Input: dimensioned drawing with shaded views. Units: mm. Origin: part minimum x, y, z. Give positions to 0.01 mm unless a question says otherwise; leave off trailing zeros. Write each loop counter-clockwise with the first axis right and the second up, starting at its lowest first coordinate (ties: lowest second). Pieces come first, ordered by that corner, then holes. Notation, with made-up numbers: M 89.25,-9 L 143.25,-9 A26 cw 143.25,29 Z; hole C 46,-32 d8. An arc over 180 degrees is marked long. Answer as a JSON object with one key per item and string values.
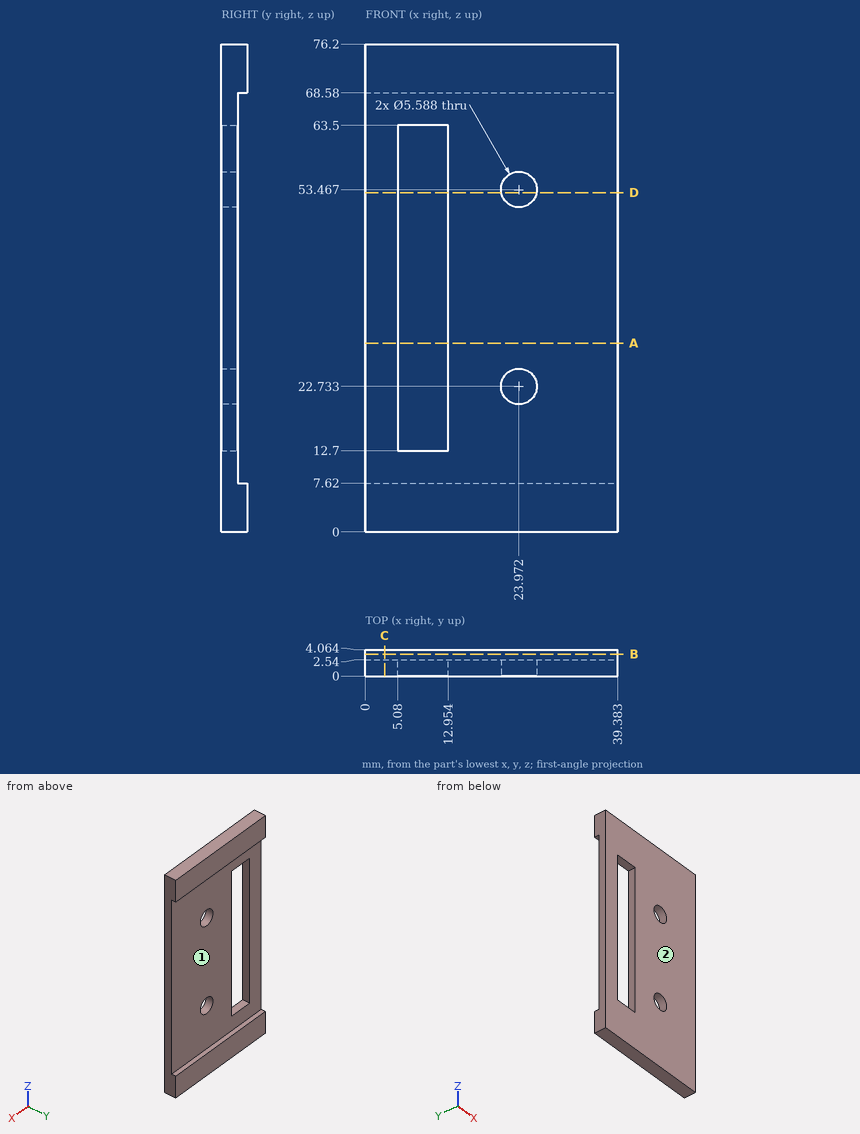
1) Cut plane D-D on z = 53. Return loops of the section in (x, y).
Geometry check:
{"outline": "M 0,0 L 5.08,0 L 5.08,2.54 L 0,2.54 Z; M 12.95,0 L 21.22,0 L 21.22,2.54 L 12.95,2.54 Z; M 26.73,0 L 39.38,0 L 39.38,2.54 L 26.73,2.54 Z"}
2) Contact query for flat-ended pins moving along their axis: P1, Ø6.5, axis at x = 23.97, z = 53.47, coming from the +Y side; P2, Ø2, axis at y = 1, z = 44, coming from the -X side. Output: stop coordinate, or through.
Geometry check:
{"P1": "stops at y = 2.54", "P2": "stops at x = 0"}
3) Pull-direction query (Z, two-part tool) for the marked faces 1 and 2; classes: pulls with the +Z half, pulls with the -Z half, needs draft (parallel to the pull), parting line crosses it, or undercut.
Geometry check:
{"face 1": "undercut", "face 2": "needs draft"}
4) Cut plane A-A on z = 29.5. Return loops of the section in (x, y).
Geometry check:
{"outline": "M 0,0 L 5.08,0 L 5.08,2.54 L 0,2.54 Z; M 12.95,0 L 39.38,0 L 39.38,2.54 L 12.95,2.54 Z"}
5) Cut plane B-B on y = 3.4. Return loops of the section in (x, z).
Geometry check:
{"outline": "M 0,0 L 39.38,0 L 39.38,7.62 L 0,7.62 Z; M 0,68.58 L 39.38,68.58 L 39.38,76.2 L 0,76.2 Z"}
6) Cut plane C-C on x = 3. Return loops of the section in (y, z).
Geometry check:
{"outline": "M 0,0 L 4.06,0 L 4.06,7.62 L 2.54,7.62 L 2.54,68.58 L 4.06,68.58 L 4.06,76.2 L 0,76.2 Z"}
7) Line query: line 1 (Z direction, x = 11, y = 0.6); line 2 (Z direction, x = 7.5, y = 3.05); line 3 (Z direction, x = 26.5, y = 1.35) (1 decimal). Output: solid intervals per line, ascending. Write a range as from..to.
Geometry check:
{"line 1": "z = 0..12.7, 63.5..76.2", "line 2": "z = 0..7.62, 68.58..76.2", "line 3": "z = 0..21.5, 23.9..52.3, 54.7..76.2"}
